Input: part model. Units: mm. Frame: model coordinates. Give positions to 0.01 mm unless a question says otherwise; leave off trailing zeros. Loops run counter-clockwise (first coordinate to the right, second up) from the corner with the lowest first, then second, coordinate; pieces in that order, holes last. Notation, with made-up numbers: (-1.75, -36.75) - (54.25, -36.75) arc R29 cw to (54.25, -9.75) - close; hole circle Ø10 at (6, 80). An arc over 180 degrees is marked (long way). Answer as a JSON object with one key per item and string values.
from build123d import *

# Parameters (mm, degrees)
BASE_EXTRUDE_DEPTH  = 2.667
SKETCH2_R           = 8.450958565
BOSS_EXTRUDE1_DEPTH = 2.667


with BuildPart() as part:
    # Sketch1 → Base-Extrude (new body)
    with BuildSketch(Plane.XY):
        with BuildLine():
            Line((6.35, -6.35), (6.35, 76.2))
            ThreePointArc((6.35, 76.2), (-179.146372853, 71.382862664), (-357.978470471, 21.873368468))
            ThreePointArc((-357.978470471, 21.873368468), (-369.761705842, 6.668454051), (-355.6, -6.35))
            Line((-355.6, -6.35), (6.35, -6.35))
        make_face()
    extrude(amount=BASE_EXTRUDE_DEPTH)

    # Sketch2 → Boss-Extrude1 (add)
    with BuildSketch(Plane.XY.offset(2.667)):
        with Locations((-262.437432145, 10.104106788)):
            Circle(SKETCH2_R)
        with Locations((-28.627578506, 20.433056145)):
            Circle(SKETCH2_R)
    extrude(amount=BOSS_EXTRUDE1_DEPTH)


solid = part.part
Item 1: Material intervals for line 1 (Z direction, x = -271, y = 28.5); line 2 (X direction, y = 13.5, z = 4.85); line 3 (X direction, y = 7, z = 1.45), sorted ascending. Write a range as [from, to].
Geometry check:
{"line 1": "z = [0, 2.67]", "line 2": "x = [-270.18, -254.7], [-33.46, -23.8]", "line 3": "x = [-369.79, 6.35]"}
Item 2: Cut plane C-C (y = 51). Return loops of the section in (x, z).
Geometry check:
{"outline": "(-273.98, 0) - (6.35, 0) - (6.35, 2.67) - (-273.98, 2.67) - close"}
Item 3: Mould query, pull axis X, two halves, no side actions, for faces 1 (the face through (-24.084, 27.559, 3.982)), 2 (the face through (-176.57, 71.763, 1.315)), 3 (the face through (-254.63, 6.87, 3.98)), 4 (the face through (-29, 21, 5.334)). Classes: released by +X, released by -X, zero draft, split by the parting line, or undercut.
Geometry check:
{"face 1": "undercut", "face 2": "split by the parting line", "face 3": "undercut", "face 4": "zero draft"}
Item 4: Cut plane B-B (x = -232). Return loops of the section in (y, z), then the cut area to 3 significant figures.
Geometry check:
{"outline": "(-6.35, 0) - (61.58, 0) - (61.58, 2.67) - (-6.35, 2.67) - close", "area": "181 mm2"}
Item 5: Contact query for a flat-ended pin moving along its axis: P1, Ø6, axis at x = -96, y = 46, coming from the +Z side. Output: stop coordinate, or through.
Geometry check:
{"P1": "stops at z = 2.67"}
Item 6: Cut plane A-A (z = 3.9). Return loops of the section in (x, y).
Geometry check:
{"outline": "circle Ø16.9 at (-262.44, 10.1); circle Ø16.9 at (-28.63, 20.43)"}
